Part model, mm, in its own coordinate system. A direction names the side the tool comes from. Give positions to 0.01 mm unless a question says otherwise; leave off trailing zeros. Write each loop counter-clockwise with the first axis right and the second up, starting at its lowest first coordinate (ties: lowest second). Pieces come first, ordered by that corner, then holes. Notation, with made-up numbers: (-32.75, 48.5) - (0.25, 48.5) arc R21 cw to (0.25, 61.5) - close; hole circle Ø6 at (87, 46.25). An arc over 180 degrees is marked (long way). Answer as a JSON object with one key per item and string values. Group by question number.
```python
from build123d import *

# Parameters (mm, degrees)
F0_W      = 9.8
F0_H      = 11.9
F1_DEPTH  = 0.8
F2_R      = 1.9
F4_DEPTH  = 6.9
F3_R      = 1.9
F5_DEPTH  = 7.7
F6_W      = 9.8
F6_H      = 0.5256494999
F7_DEPTH  = 25.4
F8_W      = 9.8
F8_H      = 0.8
F9_DEPTH  = 11.37412
F10_DEPTH = 25.4
F11_R     = 1
F13_DEPTH = 0.5


with BuildPart() as f1:
    # F0 (on Front) → F1 (new body)
    with BuildSketch(Plane.XZ):
        Rectangle(F0_W, F0_H)
    extrude(amount=F1_DEPTH)

    # F2 (on face) → F4 (join)
    with BuildSketch(Plane.XZ.offset(0.8)):
        with Locations((-1.7, -2.75)):
            Circle(F2_R)
    extrude(amount=F4_DEPTH)

    # F3 (on face) → F5 (join)
    with BuildSketch(Plane(origin=(0, 0, 0), x_dir=(-1, 0, 0), z_dir=(0, 1, 0))):
        with Locations((-1.69952, 2.74952)):
            Circle(F3_R)
    extrude(amount=-F5_DEPTH)

    # F6 (on face) → F7 (join)
    with BuildSketch(Plane.XZ.offset(0.8)):
        with Locations((0, -5.6871752501)):
            Rectangle(F6_W, F6_H)
    extrude(amount=F7_DEPTH)

    # F8 (on face) → F9 (join)
    with BuildSketch(Plane.XY.offset(-5.4243505001)):
        with Locations((0, -2.9)):
            Rectangle(F8_W, F8_H)
        with Locations((0, -7.4)):
            Rectangle(F8_W, F8_H)
    extrude(amount=F9_DEPTH)

    # F10 (cut): faces of the model
    f10_faces = [f1.faces().sort_by_distance(p)[0] for p in [
        (0, -17, -5.4243505001),
        (0, -5.15, -5.4243505001),
        (0, -1.65, -5.4243505001),
    ]]
    extrude(f10_faces, amount=-F10_DEPTH, mode=Mode.SUBTRACT)

    # F11
    f11_edges = [f1.edges().sort_by_distance(p)[0] for p in [
        (-4.9, -7.4, 5.949769),
        (-4.9, -2.9, 5.949769),
        (-4.9, -0.4, 5.95),
        (-4.9, -0.4, -5.95),
        (-4.9, -2.9, -5.95),
        (-4.9, -7.4, -5.95),
        (4.9, -7.4, 5.949769),
        (4.9, -2.9, 5.949769),
        (4.9, -0.4, 5.95),
        (4.9, -0.4, -5.95),
        (4.9, -7.4, -5.95),
        (4.9, -2.9, -5.95),
    ]]
    fillet(f11_edges, radius=F11_R)

    # F12 (on face) → F13 (join)
    with BuildSketch(Plane.XZ.offset(7.8)):
        with BuildLine():
            ThreePointArc((0, 1.95), (-1.3788989698, 1.3788174757), (-1.9499999966, -0.0001152501))
            Line((-1.9499999966, -0.0001152501), (-1.3999999953, -0.0001152501))
            ThreePointArc((-1.3999999953, -0.0001152501), (-0.9899902399, 0.9899087458), (0, 1.4))
            Line((0, 1.4), (0, 1.95))
        make_face()
        with BuildLine():
            Line((-1.3999999953, -0.0001152501), (-1.9499999966, -0.0001152501))
            ThreePointArc((-1.9499999966, -0.0001152501), (-1.3788174757, -1.3788989698), (0, -1.95))
            Line((0, -1.95), (0, -1.4))
            ThreePointArc((0, -1.4), (-0.9899087458, -0.9899902399), (-1.3999999953, -0.0001152501))
        make_face()
        with BuildLine():
            ThreePointArc((1.95, 0), (1.3788582233, 1.3788582233), (0, 1.95))
            Line((0, 1.95), (0, 1.4))
            ThreePointArc((0, 1.4), (0.9899494937, 0.9899494937), (1.4, 0))
            ThreePointArc((1.4, 0), (1.3999999988, -5.7625e-05), (1.3999999953, -0.0001152501))
            Line((1.3999999953, -0.0001152501), (1.9499999966, -0.0001152501))
            ThreePointArc((1.9499999966, -0.0001152501), (1.9499999991, -5.7625e-05), (1.95, 0))
        make_face()
        with BuildLine():
            Line((0, -1.4), (0, -1.95))
            ThreePointArc((0, -1.95), (1.3788174757, -1.3788989698), (1.9499999966, -0.0001152501))
            Line((1.9499999966, -0.0001152501), (1.3999999953, -0.0001152501))
            ThreePointArc((1.3999999953, -0.0001152501), (0.9899087458, -0.9899902399), (0, -1.4))
        make_face()
    extrude(amount=F13_DEPTH)


solid = f1.part
```
1) Saw through at D-D (z = 1.75). List the corners of the cut face in (x, y), and give its area (3 significant figures).
2) Drill centre lines: line 1 along Y through (x, z) = (-0.75, 5.25); line 2 along Y through (x, z) = (0, -3); line 3 along Z through (x, y) = (4.25, -2.75). Where is each one in solid material? Low to high. Write a range as from..to.
3) Saw through at B-B (x = 2.75). List the corners of the cut face in (y, z).
4) Saw through at C-C (y = -6.5). List the corners of the cut face in (x, z).
5) Which spindle directions (+Z, -Z, +X, -X, +Y, -Y) get a long thin tool onto all of the face, cutting with end or side? Do faces 1 (the flat face through (-2.2, -7.8, -0.1)), 2 (the flat face through (0, -0.8, 0)), 3 (the flat face through (-0.1, -7.4, -5.95)). Say none if no direction does.
6) Two-plate mould, pull along Y, no slides. Class faces 4 (the flat face through (0, -7.8, 0)), 5 (the cylindrical face through (-4.615, -2.906, -5.649)), 6 (the flat face through (0, -2.5, 0)): +Y half, -Y half, draft (parallel to the pull), parting line (faces both ways), or undercut.
7) Saw through at A-A (z = -2.75). List the corners of the cut face in (x, y).
Checks:
{
 "1": {"outline": "(-4.9, -7.8) - (-0.86, -7.8) - (-0.86, -8.3) - (0.86, -8.3) - (0.86, -7.8) - (4.9, -7.8) - (4.9, -7) - (3.32, -7) - (3.32, -3.3) - (4.9, -3.3) - (4.9, -2.5) - (3.32, -2.5) - (3.32, -0.8) - (4.9, -0.8) - (4.9, 0) - (-4.9, 0) - (-4.9, -0.8) - (0.08, -0.8) - (0.08, -2.5) - (-4.9, -2.5) - (-4.9, -3.3) - (0.08, -3.3) - (0.08, -7) - (-4.9, -7) - close", "area": "41.8 mm2"},
 "2": {"line 1": "-7.8..-7, -3.3..-2.5, -0.8..0", "line 2": "-7.8..0", "line 3": "-5.89..5.89"},
 "3": {"outline": "(-7.8, -5.95) - (-7, -5.95) - (-7, 1.17) - (-3.3, 1.17) - (-3.3, -5.95) - (-2.5, -5.95) - (-2.5, 1.17) - (-0.8, 1.17) - (-0.8, -5.95) - (0, -5.95) - (0, 5.95) - (-0.8, 5.95) - (-0.8, 4.33) - (-2.5, 4.33) - (-2.5, 5.95) - (-3.3, 5.95) - (-3.3, 4.33) - (-7, 4.33) - (-7, 5.95) - (-7.8, 5.95) - close"},
 "4": {"outline": "circle Ø3.8 at (-1.7, -2.75); circle Ø3.8 at (1.7, 2.75)"},
 "5": {"face 1": "-Y", "face 2": "none", "face 3": "-Z, +X, -X, +Y, -Y"},
 "6": {"face 4": "-Y half", "face 5": "draft", "face 6": "undercut"},
 "7": {"outline": "(-4.9, -7.8) - (4.9, -7.8) - (4.9, -7) - (0.2, -7) - (0.2, -3.3) - (4.9, -3.3) - (4.9, -2.5) - (0.2, -2.5) - (0.2, -0.8) - (4.9, -0.8) - (4.9, 0) - (-4.9, 0) - (-4.9, -0.8) - (-3.6, -0.8) - (-3.6, -2.5) - (-4.9, -2.5) - (-4.9, -3.3) - (-3.6, -3.3) - (-3.6, -7) - (-4.9, -7) - close"}
}
